```python
from build123d import *

# Parameters (mm, degrees)
BASE_DEPTH              = 3
ESQUISSE2_W             = 20
ESQUISSE2_H             = 20
ENL_V_MAT_EXTRU_1_DEPTH = 4
CONG_1_R                = 3
ESQUISSE4_R             = 1.25
ESQUISSE4_R_2           = 1.5
ENL_V_MAT_EXTRU_4_DEPTH = 4
ENL_V_MAT_EXTRU_5_REACH = 5
ESQUISSE5_R             = 2.25
ESQUISSE5_W             = 15.031140496
ESQUISSE5_H             = 52.322618027
PONT_H_MAL_PLACE_2_R    = 1.75
PONT_H_MAL_PLACE_DEPTH  = 3
ESQUISSE10_W            = 10
ESQUISSE10_H            = 3
ESQUISSE10_W_2          = 3
ESQUISSE10_H_2          = 30
ENL_V_MAT_EXTRU_7_DEPTH = 3


with BuildPart() as part:
    # Esquisse1 → Base (new body)
    with BuildSketch(Plane.XY):
        Polygon((0, 0), (-175, 0), (-199.748737342, 24.748737342), (-199.748737342, 284.748737342), (-175, 309.497474683), (0, 309.497474683), (24.748737342, 284.748737342), (24.748737342, 24.748737342), align=None)
    extrude(amount=BASE_DEPTH)

    # Esquisse2 → Enlèv. mat.-Extru.1 (cut, through all)
    with BuildSketch(Plane.XY.offset(3)):
        with Locations((-152.5, 286.497474683)):
            Rectangle(ESQUISSE2_W, ESQUISSE2_H)
        with Locations((-152.5, 23)):
            Rectangle(ESQUISSE2_W, ESQUISSE2_H)
        with Locations((-22.5, 23)):
            Rectangle(ESQUISSE2_W, ESQUISSE2_H)
        with Locations((-22.5, 286.497474683)):
            Rectangle(ESQUISSE2_W, ESQUISSE2_H)
    extrude(amount=-ENL_V_MAT_EXTRU_1_DEPTH, mode=Mode.SUBTRACT)

    # Congé1
    cong_1_edges = [part.edges().sort_by_distance(p)[0] for p in [
        (0, 0, 1.5),
        (-175, 0, 1.5),
        (-199.748737342, 24.748737342, 1.5),
        (-199.748737342, 284.748737342, 1.5),
        (-175, 309.497474683, 1.5),
        (0, 309.497474683, 1.5),
        (24.748737342, 284.748737342, 1.5),
        (24.748737342, 24.748737342, 1.5),
    ]]
    fillet(cong_1_edges, radius=CONG_1_R)

    # Esquisse4 → Enlèv. mat.-Extru.4 (cut, through all)
    with BuildSketch(Plane.XY.offset(3)):
        with Locations((-78.748737342, 98.497474683)):
            Circle(ESQUISSE4_R)
        with Locations((-127.748737342, 98.497474683)):
            Circle(ESQUISSE4_R)
        with Locations((-78.748737342, 40.497474683)):
            Circle(ESQUISSE4_R)
        with Locations((-127.748737342, 40.497474683)):
            Circle(ESQUISSE4_R)
        with Locations((-129.748737342, 185.997474683)):
            Circle(ESQUISSE4_R_2)
        with Locations((-89.248737342, 227.997474683)):
            Circle(ESQUISSE4_R_2)
        with BuildLine():
            Line((-82.748737342, 166.997474683), (-132.748737342, 166.997474683))
            ThreePointArc((-132.748737342, 166.997474683), (-134.162950904, 166.411688245), (-134.748737342, 164.997474683))
            Line((-134.748737342, 164.997474683), (-134.748737342, 148.997474683))
            ThreePointArc((-134.748737342, 148.997474683), (-134.162950904, 147.583261121), (-132.748737342, 146.997474683))
            Line((-132.748737342, 146.997474683), (-82.748737342, 146.997474683))
            ThreePointArc((-82.748737342, 146.997474683), (-81.334523779, 147.583261121), (-80.748737342, 148.997474683))
            Line((-80.748737342, 148.997474683), (-80.748737342, 164.997474683))
            ThreePointArc((-80.748737342, 164.997474683), (-81.334523779, 166.411688245), (-82.748737342, 166.997474683))
        make_face()
    extrude(amount=-ENL_V_MAT_EXTRU_4_DEPTH, mode=Mode.SUBTRACT)

    # Esquisse5 → Enlèv. mat.-Extru.5 (cut, up to next)
    with BuildSketch(Plane.XY.offset(3), mode=Mode.PRIVATE) as enl_v_mat_extru_5_sk1:
        with Locations((-111.738429941, 3.832493236)):
            Circle(ESQUISSE5_R)
    enl_v_mat_extru_5_tool1 = extrude(enl_v_mat_extru_5_sk1.sketch, amount=-ENL_V_MAT_EXTRU_5_REACH, mode=Mode.PRIVATE) & part.part
    add(enl_v_mat_extru_5_tool1.solids().sort_by_distance((-111.73843, 3.832493, 3))[0], mode=Mode.SUBTRACT)
    # Esquisse5 → Enlèv. mat.-Extru.5 (cut, up to next)
    with BuildSketch(Plane.XY.offset(3), mode=Mode.PRIVATE) as enl_v_mat_extru_5_sk2:
        with Locations((-89.268885084, 3.53845203)):
            Circle(ESQUISSE5_R)
    enl_v_mat_extru_5_tool2 = extrude(enl_v_mat_extru_5_sk2.sketch, amount=-ENL_V_MAT_EXTRU_5_REACH, mode=Mode.PRIVATE) & part.part
    add(enl_v_mat_extru_5_tool2.solids().sort_by_distance((-89.268885, 3.538452, 3))[0], mode=Mode.SUBTRACT)
    # Esquisse5 → Enlèv. mat.-Extru.5 (cut, up to next)
    with BuildSketch(Plane.XY.offset(3), mode=Mode.PRIVATE) as enl_v_mat_extru_5_sk3:
        with Locations((-89.268885084, 33.46154797)):
            Circle(ESQUISSE5_R)
    enl_v_mat_extru_5_tool3 = extrude(enl_v_mat_extru_5_sk3.sketch, amount=-ENL_V_MAT_EXTRU_5_REACH, mode=Mode.PRIVATE) & part.part
    add(enl_v_mat_extru_5_tool3.solids().sort_by_distance((-89.268885, 33.461548, 3))[0], mode=Mode.SUBTRACT)
    # Esquisse5 → Enlèv. mat.-Extru.5 (cut, up to next)
    with BuildSketch(Plane.XY.offset(3), mode=Mode.PRIVATE) as enl_v_mat_extru_5_sk4:
        with Locations((-111.738429941, 33.167506764)):
            Circle(ESQUISSE5_R)
    enl_v_mat_extru_5_tool4 = extrude(enl_v_mat_extru_5_sk4.sketch, amount=-ENL_V_MAT_EXTRU_5_REACH, mode=Mode.PRIVATE) & part.part
    add(enl_v_mat_extru_5_tool4.solids().sort_by_distance((-111.73843, 33.167507, 3))[0], mode=Mode.SUBTRACT)
    # Esquisse5 → Enlèv. mat.-Extru.5 (cut, up to next)
    with BuildSketch(Plane.XY.offset(3), mode=Mode.PRIVATE) as enl_v_mat_extru_5_sk5:
        with Locations((-49.05, 12.640927164)):
            Circle(ESQUISSE5_R)
    enl_v_mat_extru_5_tool5 = extrude(enl_v_mat_extru_5_sk5.sketch, amount=-ENL_V_MAT_EXTRU_5_REACH, mode=Mode.PRIVATE) & part.part
    add(enl_v_mat_extru_5_tool5.solids().sort_by_distance((-49.05, 12.640927, 3))[0], mode=Mode.SUBTRACT)
    # Esquisse5 → Enlèv. mat.-Extru.5 (cut, up to next)
    with BuildSketch(Plane.XY.offset(3), mode=Mode.PRIVATE) as enl_v_mat_extru_5_sk6:
        with Locations((-13.95, 9.5)):
            Circle(ESQUISSE5_R)
    enl_v_mat_extru_5_tool6 = extrude(enl_v_mat_extru_5_sk6.sketch, amount=-ENL_V_MAT_EXTRU_5_REACH, mode=Mode.PRIVATE) & part.part
    add(enl_v_mat_extru_5_tool6.solids().sort_by_distance((-13.95, 9.5, 3))[0], mode=Mode.SUBTRACT)
    # Esquisse5 → Enlèv. mat.-Extru.5 (cut, up to next)
    with BuildSketch(Plane.XY.offset(3), mode=Mode.PRIVATE) as enl_v_mat_extru_5_sk7:
        with Locations((-49.05, 59.140927164)):
            Circle(ESQUISSE5_R)
    enl_v_mat_extru_5_tool7 = extrude(enl_v_mat_extru_5_sk7.sketch, amount=-ENL_V_MAT_EXTRU_5_REACH, mode=Mode.PRIVATE) & part.part
    add(enl_v_mat_extru_5_tool7.solids().sort_by_distance((-49.05, 59.140927, 3))[0], mode=Mode.SUBTRACT)
    # Esquisse5 → Enlèv. mat.-Extru.5 (cut, up to next)
    with BuildSketch(Plane.XY.offset(3), mode=Mode.PRIVATE) as enl_v_mat_extru_5_sk8:
        with Locations((-13.95, 61.981854328)):
            Circle(ESQUISSE5_R)
    enl_v_mat_extru_5_tool8 = extrude(enl_v_mat_extru_5_sk8.sketch, amount=-ENL_V_MAT_EXTRU_5_REACH, mode=Mode.PRIVATE) & part.part
    add(enl_v_mat_extru_5_tool8.solids().sort_by_distance((-13.95, 61.981854, 3))[0], mode=Mode.SUBTRACT)
    # Esquisse5 → Enlèv. mat.-Extru.5 (cut, up to next)
    with BuildSketch(Plane.XY.offset(3), mode=Mode.PRIVATE) as enl_v_mat_extru_5_sk9:
        with Locations((8.748737342, 201.897474683)):
            Circle(ESQUISSE5_R)
    enl_v_mat_extru_5_tool9 = extrude(enl_v_mat_extru_5_sk9.sketch, amount=-ENL_V_MAT_EXTRU_5_REACH, mode=Mode.PRIVATE) & part.part
    add(enl_v_mat_extru_5_tool9.solids().sort_by_distance((8.748737, 201.897475, 3))[0], mode=Mode.SUBTRACT)
    # Esquisse5 → Enlèv. mat.-Extru.5 (cut, up to next)
    with BuildSketch(Plane.XY.offset(3), mode=Mode.PRIVATE) as enl_v_mat_extru_5_sk10:
        with Locations((11.889664506, 236.997474683)):
            Circle(ESQUISSE5_R)
    enl_v_mat_extru_5_tool10 = extrude(enl_v_mat_extru_5_sk10.sketch, amount=-ENL_V_MAT_EXTRU_5_REACH, mode=Mode.PRIVATE) & part.part
    add(enl_v_mat_extru_5_tool10.solids().sort_by_distance((11.889665, 236.997475, 3))[0], mode=Mode.SUBTRACT)
    # Esquisse5 → Enlèv. mat.-Extru.5 (cut, up to next)
    with BuildSketch(Plane.XY.offset(3), mode=Mode.PRIVATE) as enl_v_mat_extru_5_sk11:
        with Locations((-37.751262658, 201.897474683)):
            Circle(ESQUISSE5_R)
    enl_v_mat_extru_5_tool11 = extrude(enl_v_mat_extru_5_sk11.sketch, amount=-ENL_V_MAT_EXTRU_5_REACH, mode=Mode.PRIVATE) & part.part
    add(enl_v_mat_extru_5_tool11.solids().sort_by_distance((-37.751263, 201.897475, 3))[0], mode=Mode.SUBTRACT)
    # Esquisse5 → Enlèv. mat.-Extru.5 (cut, up to next)
    with BuildSketch(Plane.XY.offset(3), mode=Mode.PRIVATE) as enl_v_mat_extru_5_sk12:
        with Locations((-40.592189823, 236.997474683)):
            Circle(ESQUISSE5_R)
    enl_v_mat_extru_5_tool12 = extrude(enl_v_mat_extru_5_sk12.sketch, amount=-ENL_V_MAT_EXTRU_5_REACH, mode=Mode.PRIVATE) & part.part
    add(enl_v_mat_extru_5_tool12.solids().sort_by_distance((-40.59219, 236.997475, 3))[0], mode=Mode.SUBTRACT)
    # Esquisse5 → Enlèv. mat.-Extru.5 (cut, up to next)
    with BuildSketch(Plane.XY.offset(3), mode=Mode.PRIVATE) as enl_v_mat_extru_5_sk13:
        with Locations((-18.655958793, 109.451399186)):
            Circle(ESQUISSE5_R)
    enl_v_mat_extru_5_tool13 = extrude(enl_v_mat_extru_5_sk13.sketch, amount=-ENL_V_MAT_EXTRU_5_REACH, mode=Mode.PRIVATE) & part.part
    add(enl_v_mat_extru_5_tool13.solids().sort_by_distance((-18.655959, 109.451399, 3))[0], mode=Mode.SUBTRACT)
    # Esquisse5 → Enlèv. mat.-Extru.5 (cut, up to next)
    with BuildSketch(Plane.XY.offset(3), mode=Mode.PRIVATE) as enl_v_mat_extru_5_sk14:
        with Locations((-18.95, 86.981854328)):
            Circle(ESQUISSE5_R)
    enl_v_mat_extru_5_tool14 = extrude(enl_v_mat_extru_5_sk14.sketch, amount=-ENL_V_MAT_EXTRU_5_REACH, mode=Mode.PRIVATE) & part.part
    add(enl_v_mat_extru_5_tool14.solids().sort_by_distance((-18.95, 86.981854, 3))[0], mode=Mode.SUBTRACT)
    # Esquisse5 → Enlèv. mat.-Extru.5 (cut, up to next)
    with BuildSketch(Plane.XY.offset(3), mode=Mode.PRIVATE) as enl_v_mat_extru_5_sk15:
        with Locations((10.973095941, 86.981854328)):
            Circle(ESQUISSE5_R)
    enl_v_mat_extru_5_tool15 = extrude(enl_v_mat_extru_5_sk15.sketch, amount=-ENL_V_MAT_EXTRU_5_REACH, mode=Mode.PRIVATE) & part.part
    add(enl_v_mat_extru_5_tool15.solids().sort_by_distance((10.973096, 86.981854, 3))[0], mode=Mode.SUBTRACT)
    # Esquisse5 → Enlèv. mat.-Extru.5 (cut, up to next)
    with BuildSketch(Plane.XY.offset(3), mode=Mode.PRIVATE) as enl_v_mat_extru_5_sk16:
        with Locations((10.679054734, 109.451399186)):
            Circle(ESQUISSE5_R)
    enl_v_mat_extru_5_tool16 = extrude(enl_v_mat_extru_5_sk16.sketch, amount=-ENL_V_MAT_EXTRU_5_REACH, mode=Mode.PRIVATE) & part.part
    add(enl_v_mat_extru_5_tool16.solids().sort_by_distance((10.679055, 109.451399, 3))[0], mode=Mode.SUBTRACT)
    # Esquisse5 → Enlèv. mat.-Extru.5 (cut, up to next)
    with BuildSketch(Plane.XY.offset(3), mode=Mode.PRIVATE) as enl_v_mat_extru_5_sk17:
        with Locations((-60.577832016, 26.161309014)):
            Rectangle(ESQUISSE5_W, ESQUISSE5_H)
    enl_v_mat_extru_5_tool17 = extrude(enl_v_mat_extru_5_sk17.sketch, amount=-ENL_V_MAT_EXTRU_5_REACH, mode=Mode.PRIVATE) & part.part
    add(enl_v_mat_extru_5_tool17.solids().sort_by_distance((-60.577832, 26.161309, 3))[0], mode=Mode.SUBTRACT)

    # PONT H mal place 2 → pont_H_mal_place (cut)
    with BuildSketch(Plane.XY.offset(3)):
        with Locations((-69.262539319, 120.947398703)):
            Circle(PONT_H_MAL_PLACE_2_R)
        with Locations((-69.262539319, 84.205598383)):
            Circle(PONT_H_MAL_PLACE_2_R)
        with Locations((-31.776164099, 84.205598383)):
            Circle(PONT_H_MAL_PLACE_2_R)
        with Locations((-31.776164099, 120.947398703)):
            Circle(PONT_H_MAL_PLACE_2_R)
    extrude(amount=-PONT_H_MAL_PLACE_DEPTH, mode=Mode.SUBTRACT)

    # Esquisse10 → Enlèv. mat.-Extru.7 (cut)
    with BuildSketch(Plane.XY.offset(3)):
        with Locations((-176.748737342, 58.248737342)):
            Rectangle(ESQUISSE10_W, ESQUISSE10_H)
        with Locations((-188.248737342, 95.748737342)):
            Rectangle(ESQUISSE10_W_2, ESQUISSE10_H_2)
        with Locations((-156.748737342, 58.248737342)):
            Rectangle(ESQUISSE10_W, ESQUISSE10_H)
        with Locations((-145.248737342, 95.748737342)):
            Rectangle(ESQUISSE10_W_2, ESQUISSE10_H_2)
        with Locations((-188.248737342, 173.748737342)):
            Rectangle(ESQUISSE10_W_2, ESQUISSE10_H_2)
        with Locations((-156.748737342, 211.248737342)):
            Rectangle(ESQUISSE10_W, ESQUISSE10_H)
        with Locations((-176.748737342, 211.248737342)):
            Rectangle(ESQUISSE10_W, ESQUISSE10_H)
        with Locations((-145.248737342, 173.748737342)):
            Rectangle(ESQUISSE10_W_2, ESQUISSE10_H_2)
    extrude(amount=-ENL_V_MAT_EXTRU_7_DEPTH, mode=Mode.SUBTRACT)


solid = part.part
```
Source: CAD feature listing. Evaluate the final solid. Frame: model axes, mm. Round coordinates to 2 decimals unless told otherwise and drop trailing zeros.
(1) Material intervals for probe 1 along Y at (x, z) = (-156, 0.6); probe 2 along X at (y, z) = (165, 2.25); probe 3 along Y at (x, z) = (-147, 0.9), sorted ascending.
From the geometry:
probe 1: y = 0 to 13, 33 to 56.75, 59.75 to 209.75, 212.75 to 276.5, 296.5 to 309.5
probe 2: x = -199.75 to -189.75, -186.75 to -146.75, -143.75 to -134.75, -80.75 to 24.75
probe 3: y = 0 to 13, 33 to 276.5, 296.5 to 309.5
(2) Contact query for flat-ended pins moving along their axis: pin 1 Ø1.5 at (x, z) = (-188, 1) entering from -Y; pin 2 Ø4 at (x, y) = (10.68, 109.45) entering from -Z. Output: stop coordinate, or through.
From the geometry:
pin 1: stops at y = 12.25
pin 2: passes through
(3) Section query A-A (z = 1.1). Give the number of separate pieces and of enclosed holes in the cut face, and give its area (3 significant figures).
From the geometry:
separate pieces: 1
enclosed holes: 39
area: 64,000 mm2
